Autodesk Inventor part; units mm, degrees
ref_plane "YZ Plane" through (0, 0, 0) normal (1, 0, 0) x (0, 1, 0)
ref_plane "XZ Plane" through (0, 0, 0) normal (0, 1, 0) x (-1, 0, 0)
ref_plane "XY Plane" through (0, 0, 0) normal (0, 0, 1) x (1, 0, 0)
sketch "Szkic1" plane through (0, 0, 0) normal (0, 1, 0) x (-1, 0, 0)
  line L0 (-25, -25) -> (25, -25)
  line L1 (25, -25) -> (25, 25)
  line L2 (-25, 25) -> (-25, -25)
  line L3 (-25, -25) -> (25, 25) construction
  line L4 (25, -25) -> (-25, 25) construction
  line L5 (10, 25) -> (-10, 25)
  line L6 (-10, 25) -> (-10, 15)
  line L7 (-10, 15) -> (10, 15)
  line L8 (10, 15) -> (10, 25)
  line L9 (-15, -10) -> (-15, 10)
  line L10 (-15, 10) -> (-25, 10)
  line L11 (-25, -10) -> (-15, -10)
  line L12 (10, -15) -> (-10, -15)
  line L13 (-10, -15) -> (-10, -25)
  line L14 (10, -25) -> (10, -15)
  line L15 (15, 10) -> (15, -10)
  line L16 (15, -10) -> (25, -10)
  line L17 (25, 10) -> (15, 10)
  line L18 (25, 25) -> (10, 25)
  line L19 (-10, 25) -> (-25, 25)
  point P0 (0, 0)
  dimension "d0" = 50
  dimension "d1" = 50
  dimension "d3" = 10
  dimension "d7" = 360
extrude "Wyciągnięcie proste1" add sketch "Szkic1" along normal blind 500 contours L2 L11 L9 L10 L19 L6 L7 L8 L18 L1 L17 L15 L16 L0 L14 L12 L13
properties part number "wysiegnik2" material "Aluminium 6061"
Geometry: final body of the model. Coordinates: model frame, mm. A direction names the side the tool comes from. Round coordinates to 2 decimals unless told otherwise and drop trailing zeros. Order: outer loops, then holes, each group sorted by start corner. A loop starts at its lowest first (then second) coordinate and runs counter-clockwise, first axis right, second up. Notation, with made-up numbers: M 39.5,-31.75 L 74.5,-31.75 A31 ccw 74.5,7.25 Z; hole C 47,-23 d9. An arc over 180 degrees is marked long. Use one line per item in the form item = value. Start each with the question number.
Q1. Mould query, pull axis Z, two halves, no side actions, for faces 1 (the face through (20, 246, -10)), 2 (the face through (-10, 246, -20)), 3 (the face through (0, 246, -15)). Classes: +Z half, -Z half, draft (parallel to the pull), parting line (faces both ways), or undercut.
Q2. Cut plane A-A (x = 20). Return loops of the section in (y, z), and give its area (3 significant figures).
Q3. Cut plane B-B (y = 95). Return loops of the section in (x, z).
Q4. Access query for faces 4 (the face through (10, 246, 20)), 5 (the face through (-15, 246, 0)), 6 (the face through (10, 246, -20)). Directions: +Z, -Z, +X, -X, +Y, -Y. A direction counts if a zero-diameter tool reaches every point of the face in a straight line with its end or side. Return the directions, or none.
Q5. Pin query (flat end, axial travel): pin 1 Ø6 at (y, z) = (262, 3.5) entering from -X; pin 2 Ø10 at (x, y) = (-4.5, 297.5) entering from +Z; pin 3 Ø1.5 at (x, y) = (7.5, 94.5) entering from -Z. Return the tip coordinate at first contact, or that it passes through.
Q6. Cut plane C-C (z = 4). Return loops of the section in (x, y).
Q7. Material intervals for line 1 (Z direction, x = -17.5, y = 228); line 2 (Z direction, x = 3.5, y = 144), sorted ascending. Write a range as [from, to].
Geometry results:
q1.face_1 = undercut
q1.face_2 = draft
q1.face_3 = -Z half
q2.outline = M 0,-25 L 500,-25 L 500,-10 L 0,-10 Z; M 0,10 L 500,10 L 500,25 L 0,25 Z
q2.area = 15,000 mm^2
q3.outline = M -25,-25 L -10,-25 L -10,-15 L 10,-15 L 10,-25 L 25,-25 L 25,-10 L 15,-10 L 15,10 L 25,10 L 25,25 L 10,25 L 10,15 L -10,15 L -10,25 L -25,25 L -25,10 L -15,10 L -15,-10 L -25,-10 Z
q4.face_4 = +Z, +Y, -Y
q4.face_5 = -X, +Y, -Y
q4.face_6 = -Z, +Y, -Y
q5.pin_1 = -15
q5.pin_2 = 15
q5.pin_3 = -15
q6.outline = M -15,0 L 15,0 L 15,500 L -15,500 Z
q7.line_1 = [-25, -10], [10, 25]
q7.line_2 = [-15, 15]
